Autodesk Inventor part; units mm, degrees
ref_plane "Work Plane1" through (29.4, -17.23, 0) normal (0, -1, 0) x (1, 0, 0)
ref_plane "YZ Plane" through (0, 0, 0) normal (1, 0, 0) x (0, 1, 0)
ref_plane "XZ Plane" through (0, 0, 0) normal (0, 1, 0) x (-1, 0, 0)
sketch "Sketch1" plane through (0, 0, 0) normal (0, 0, 1) x (1, 0, 0)
  line L0 (-29.4, -18.5) -> (29.4, -18.5)
  line L1 (29.4, -18.5) -> (29.4, 18.5)
  line L2 (29.4, 18.5) -> (-29.4, 18.5)
  line L3 (-29.4, 18.5) -> (-29.4, -18.5)
  line L4 (-29.4, -18.5) -> (29.4, 18.5) construction
  line L5 (29.4, -18.5) -> (-29.4, 18.5) construction
  point P0 (0, 0)
  dimension "d0" = 58.8
  dimension "d1" = 37
extrude "Extrusion1" add sketch "Sketch1" along normal blind 173
sketch "Sketch2" plane through (-29.4, 18.5, 0) normal (0, 1, 0) x (1, 0, 0)
  line L0 (58.8, -173) -> (0, -173)
  line L1 (58.8, 0) -> (0, 0)
  arc A0 (22.65, -167.5) -> (18.15, -167.5) centre (20.4, -167.5) ccw
  arc A1 (40.65, -167.5) -> (36.15, -167.5) centre (38.4, -167.5) ccw
  arc A2 (36.15, -5.5) -> (40.65, -5.5) centre (38.4, -5.5) ccw
  arc A3 (18.15, -5.5) -> (22.65, -5.5) centre (20.4, -5.5) ccw
  line L2 (20.4, -167.5) -> (20.4, -5.5) construction
  line L3 (20.4, -5.5) -> (38.4, -5.5) construction
  line L4 (38.4, -5.5) -> (38.4, -167.5) construction
  line L5 (20.4, -167.5) -> (20.4, -173) construction
  line L6 (20.4, -5.5) -> (20.4, 0) construction
  line L7 (20.4, -5.5) -> (0, 0) construction
  line L8 (38.4, -5.5) -> (58.8, 0) construction
  line L9 (36.15, -167.5) -> (36.15, -173)
  line L10 (40.65, -167.5) -> (40.65, -173)
  line L11 (18.15, -167.5) -> (18.15, -173)
  line L12 (22.65, -167.5) -> (22.65, -173)
  line L13 (22.65, -5.5) -> (22.65, 0)
  line L14 (18.15, -5.5) -> (18.15, 0)
  line L15 (40.65, -5.5) -> (40.65, 0)
  line L16 (36.15, -5.5) -> (36.15, 0)
  point P0 (29.4, 0)
  dimension "d4" = 2.25
  dimension "d5" = 162
  dimension "d6" = 18
extrude "Extrusion2" cut sketch "Sketch2" against normal up to surface (37 mm away)
ref_plane "Work Plane1" through (29.4, -17.23, 0) normal (0, -1, 0) x (1, 0, 0)
sketch "Sketch3" plane through (-29.4, 18.5, 173) normal (0, 1, 0) x (1, 0, 0)
  line L0 (0, 173) -> (0, 0)
  line L1 (58.8, 173) -> (58.8, 0)
  line L2 (57.53, 0) -> (57.53, 10.5)
  line L3 (57.53, 10.5) -> (1.27, 10.5)
  line L4 (1.27, 10.5) -> (1.27, 0)
  line L5 (1.27, 0) -> (57.53, 0)
  line L6 (1.27, 0) -> (0, 0) construction
  line L7 (58.8, 0) -> (57.53, 0) construction
  line L8 (1.27, 162.5) -> (57.53, 162.5)
  line L9 (57.53, 162.5) -> (57.53, 173)
  line L10 (57.53, 173) -> (1.27, 173)
  line L11 (1.27, 173) -> (1.27, 162.5)
  line L12 (1.27, 173) -> (0, 173) construction
  point P0 (29.4, 173)
  dimension "d9" = 1.27
  dimension "d14" = 152
extrude "Extrusion3" cut sketch "Sketch3" against normal up to surface (35.73 mm away)
properties part number "UHP-1500-230"
The listing builds one solid part. Answer for the finished solid, in the listing's coordinates (mm). A direction names the side the tool comes from. Round coordinates to 2 decimals unless told otherwise and drop trailing zeros. Order: outer loops, then holes, each group sorted by start corner. A loop starts at its lowest first (then second) coordinate and runs counter-clockwise, first axis right, second up. Notation, with made-up numbers: (3, -12.75) -> (24, -12.75) arc R12 ccw to (24, 6.25) -> close; hole circle Ø5 at (19, 81). An arc over 180 degrees is marked (long way). Write each question's results on one line, items separated by ' | '. Start each with the question number.
Q1. A straight line is drawn through the part: probe 1 along Z at (x, y) = (-24.5, 6). Find the intervals that lie inside material, in ascending order. Write a range as from..to.
Q2. Find section C-C (x = -16.5). Determine the outline of the cut face in (y, z), then the cut area to 3 significant figures.
Q3. Find section A-A (y = 12). Determine the outline of the cut face in (x, z).
Q4. Which of the six approach directions +Z, -Z, +X, -X, +Y, -Y give full straight-line access (tool end or side, diameter ignored) to faces 1 (the flat face through (-28.13, 1, 168)), 2 (the flat face through (0, 18.5, 85)), 3 (the flat face through (0, 1, 10.5))?
Q5. Each of these flat-tipped pins is pushed along its axis until it touches: pin 1 (18 mm diameter, centred on x = -6, y = -3, fed in from +Z); pin 2 (3 mm diameter, centred on x = -10, z = 165, fed in from +Y); pin 3 (3 mm diameter, centred on x = 23.5, y = 0.5, fed in from -Z). Where does it stop, or does it pass through?
Q6. Find section B-B (x = -9). Determine the outline of the cut face in (y, z).
Q7. The mould has two halves that part along X. Classify faces 4 (the flat face through (0, -18.5, 85)), 5 (the flat face through (28.13, 1, 5)), 6 (the flat face through (-29.4, 0, 85)): pulls with the +X half, pulls with the -X half, needs draft (parallel to the pull), parting line crosses it, or undercut.
Worked answers:
1) probe 1: z = 10.5..162.5
2) outline: (-18.5, 0) -> (-17.23, 0) -> (-17.23, 10.5) -> (18.5, 10.5) -> (18.5, 162.5) -> (-17.23, 162.5) -> (-17.23, 173) -> (-18.5, 173) -> close | area: 5,650 mm2
3) outline: (-29.4, 0) -> (-28.13, 0) -> (-28.13, 10.5) -> (28.13, 10.5) -> (28.13, 0) -> (29.4, 0) -> (29.4, 173) -> (28.13, 173) -> (28.13, 162.5) -> (-28.13, 162.5) -> (-28.13, 173) -> (-29.4, 173) -> close
4) face 1: +Z, +Y | face 2: +Z, -Z, +X, -X, +Y | face 3: -Z, +Y
5) pin 1: stops at z = 162.5 | pin 2: stops at y = -17.23 | pin 3: stops at z = 10.5
6) outline: (-18.5, 7.75) -> (-17.23, 7.75) -> (-17.23, 10.5) -> (18.5, 10.5) -> (18.5, 162.5) -> (-17.23, 162.5) -> (-17.23, 165.25) -> (-18.5, 165.25) -> close
7) face 4: needs draft | face 5: undercut | face 6: pulls with the -X half
